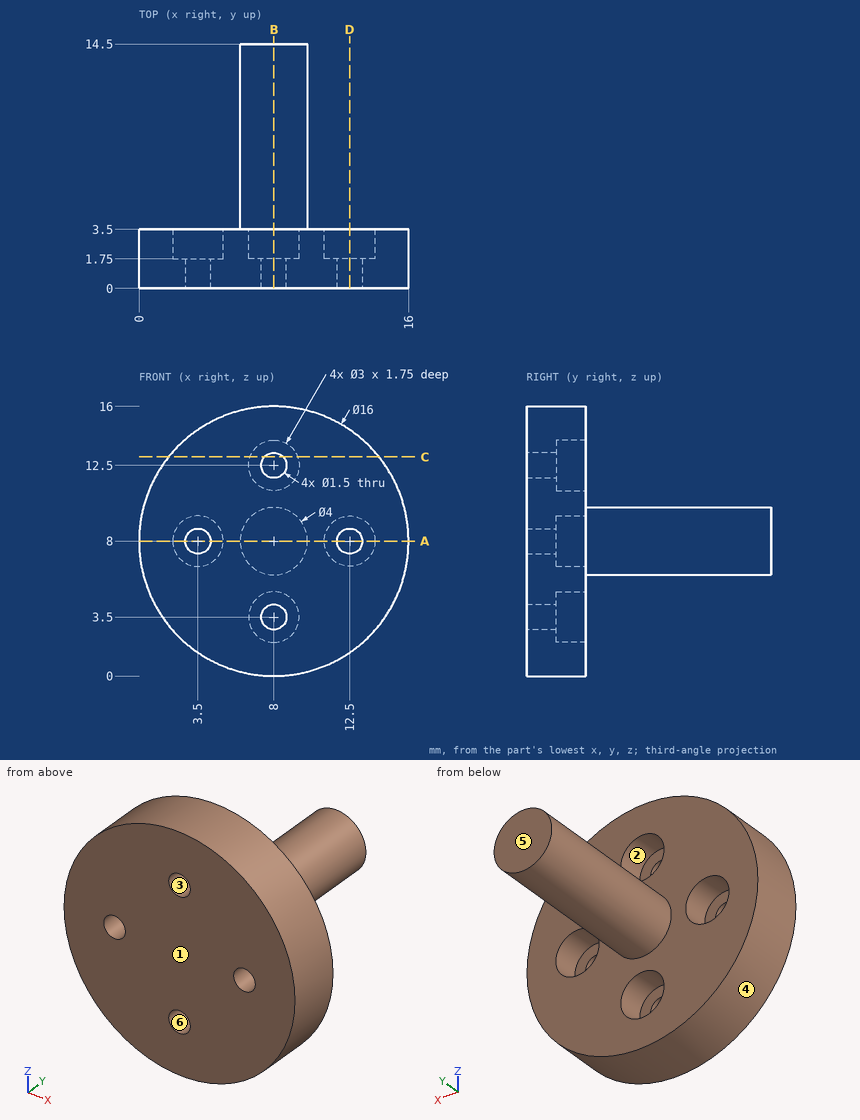
Check sheet for the drawn part. Datum: minimum x, y, z corner. Units: mm. A direction names the side the tool comes from. Round coordinates to 2 decimals unless told otherwise and drop trailing zeros. Loops run counter-clockwise (first coordinate to the right, second up) from the corner with the lowest first, then second, coordinate; pieces in that order, holes last.
Item 1: Cross-section at A-A on z = 8. Record the boundary of the cut face in (x, y).
Item 2: Gauge pin test, flat ends, axial feed: pin 1 (4 mm diameter, centred on y = 8.5, z = 7.5, fed in from -X); pin 2 (0.9 mm diameter, centred on x = 13, z = 8, fed in from +Y); pin 3 (3.5 mm diameter, centred on x = 8, z = 12.5, fed in from +Y). Record the tip position at first contact, or that the pin passes through.
Item 3: Cross-section at C-C on z = 13. Record the boundary of the cut face in (x, y) (3 decimals).
Item 4: Cross-section at D-D on x = 12.5. Record the boundary of the cut face in (y, z).
Item 5: Cross-section at B-B on x = 8. Record the boundary of the cut face in (y, z), then the cut area to 4 significant figures.
Item 6: Access from +Z, -Z, +X, -X, +Y, -Y to the whole of each face (thin tool, end or side, straight path). Record for the marked faces 1 and 2.
Item 7: Thickness scan on line 1 (Z direction, x = 8, y = 2.3); line 2 (Y direction, x = 12.25, z = 5); line 3 (Y direction, x = 7.5, z = 4.5). Record the ranges inside material, lowest first.
Item 8: Mould release check, pull along X, two halves, no side actions. Record for the marked faces 3, 4, 5 and 6: pulls with the +X half, pulls with the -X half, needs draft (parallel to the pull), parting line crosses it, or undercut.
Answer sheet:
1. outline: (0, 0) - (2.75, 0) - (2.75, 1.75) - (2, 1.75) - (2, 3.5) - (0, 3.5) - close; (4.25, 0) - (11.75, 0) - (11.75, 1.75) - (11, 1.75) - (11, 3.5) - (10, 3.5) - (10, 14.5) - (6, 14.5) - (6, 3.5) - (5, 3.5) - (5, 1.75) - (4.25, 1.75) - close; (13.25, 0) - (16, 0) - (16, 3.5) - (14, 3.5) - (14, 1.75) - (13.25, 1.75) - close
2. pin 1: stops at x = 6
2. pin 2: stops at y = 1.75
2. pin 3: stops at y = 3.5
3. outline: (1.755, 0) - (7.441, 0) - (7.441, 1.75) - (6.586, 1.75) - (6.586, 3.5) - (1.755, 3.5) - close; (8.559, 0) - (14.245, 0) - (14.245, 3.5) - (9.414, 3.5) - (9.414, 1.75) - (8.559, 1.75) - close
4. outline: (0, 1.39) - (3.5, 1.39) - (3.5, 6.5) - (1.75, 6.5) - (1.75, 7.25) - (0, 7.25) - close; (0, 8.75) - (1.75, 8.75) - (1.75, 9.5) - (3.5, 9.5) - (3.5, 14.61) - (0, 14.61) - close
5. outline: (0, 0) - (3.5, 0) - (3.5, 2) - (1.75, 2) - (1.75, 2.75) - (0, 2.75) - close; (0, 4.25) - (1.75, 4.25) - (1.75, 5) - (3.5, 5) - (3.5, 6) - (14.5, 6) - (14.5, 10) - (3.5, 10) - (3.5, 11) - (1.75, 11) - (1.75, 11.75) - (0, 11.75) - close; (0, 13.25) - (1.75, 13.25) - (1.75, 14) - (3.5, 14) - (3.5, 16) - (0, 16) - close
5. area: 84.25 mm2
6. face 1: +Z, -Z, +X, -X, -Y
6. face 2: +Y
7. line 1: z = 0 to 2, 5 to 11, 14 to 16
7. line 2: y = 0 to 3.5
7. line 3: y = 0 to 1.75
8. face 3: undercut
8. face 4: parting line crosses it
8. face 5: needs draft
8. face 6: undercut
